```python
from build123d import *

# Parameters (mm, degrees)
BOSS_EXTRUDE1_DEPTH                     = 1247.2780762
BOSS_EXTRUDE1_DEPTH_BACK                = 0.0001
CBORE_FOR_M5_HEX_HEAD_BOLT1_D           = 5.8
CBORE_FOR_M5_HEX_HEAD_BOLT1_CBORE_D     = 12.238
CBORE_FOR_M5_HEX_HEAD_BOLT1_CBORE_DEPTH = 3.5
SKETCH12_R                              = 2.192561761
SKETCH12_R_2                            = 2.198183891
SKETCH12_R_3                            = 2.178555517
SKETCH12_R_4                            = 2.1825859
SKETCH12_R_5                            = 2.191093622
SKETCH12_R_6                            = 2.184131757
SKETCH12_W                              = 20.639060425
SKETCH12_H                              = 4.385123522
SKETCH12_W_2                            = 20.62721893
CUT_EXTRUDE3_DEPTH                      = 219
SCALE1_SCALE                            = 1.8


with BuildPart() as part:
    # Sketch1 → Boss-Extrude1 (new, two sides: drawn at the far end of the back side and taken through both)
    with BuildSketch(Plane.XY.offset(-BOSS_EXTRUDE1_DEPTH_BACK)):
        Polygon((-11.227272727, -5.287267028), (10.772727273, -5.287267028), (10.772727273, 1.712732972), (12.272727273, 1.712732972), (12.272727273, -6.687267028), (-12.727272727, -6.687267028), (-12.727272727, 1.712732972), (-11.227272727, 1.712732972), align=None)
    extrude(amount=BOSS_EXTRUDE1_DEPTH + BOSS_EXTRUDE1_DEPTH_BACK)

    # CBORE for M5 Hex Head Bolt1 (through all)
    with Locations(Plane(origin=(0, -5.287267028, 0), x_dir=(1, 0, 0), z_dir=(0, 1, 0))):
        with Locations((0, -26.226555277), (0, -53.601555277), (0, -80.976555277), (0, -108.351555277), (0, -135.726555277), (0, -163.101555277), (0, -190.476555277), (0, -217.851555277)):
            CounterBoreHole(CBORE_FOR_M5_HEX_HEAD_BOLT1_D / 2, CBORE_FOR_M5_HEX_HEAD_BOLT1_CBORE_D / 2, CBORE_FOR_M5_HEX_HEAD_BOLT1_CBORE_DEPTH)

    # Sketch12 → Cut-Extrude3 (cut)
    with BuildSketch(Plane.ZY.offset(12.727272727)):
        with Locations((13.543356252, -2.543007858)):
            Circle(SKETCH12_R)
        with Locations((34.182416677, -2.543007858)):
            Circle(SKETCH12_R_2)
        with Locations((65.305213992, -2.710382167)):
            Circle(SKETCH12_R)
        with Locations((85.932432922, -2.710382167)):
            Circle(SKETCH12_R_3)
        with Locations((112.703179644, -2.640183104)):
            Circle(SKETCH12_R)
        with Locations((133.330398574, -2.640183104)):
            Circle(SKETCH12_R_4)
        with Locations((164.345985992, -2.803798306)):
            Circle(SKETCH12_R)
        with Locations((184.973204922, -2.803798306)):
            Circle(SKETCH12_R_5)
        with Locations((216.107843732, -2.971172615)):
            Circle(SKETCH12_R)
        with Locations((236.735062662, -2.971172615)):
            Circle(SKETCH12_R_6)
        with Locations((23.862886465, -2.543007858)):
            Rectangle(SKETCH12_W, SKETCH12_H)
        with Locations((75.618823457, -2.710382167)):
            Rectangle(SKETCH12_W_2, SKETCH12_H)
        with Locations((123.016789109, -2.640183104)):
            Rectangle(SKETCH12_W_2, SKETCH12_H)
        with Locations((174.659595457, -2.803798306)):
            Rectangle(SKETCH12_W_2, SKETCH12_H)
        with Locations((226.421453197, -2.971172615)):
            Rectangle(SKETCH12_W_2, SKETCH12_H)
    extrude(amount=-CUT_EXTRUDE3_DEPTH, mode=Mode.SUBTRACT)


with BuildPart() as part_1:
    # Scale1: scaled about (0, 0, 0)
    add(part.part.scale(SCALE1_SCALE))


solid = part_1.part
```
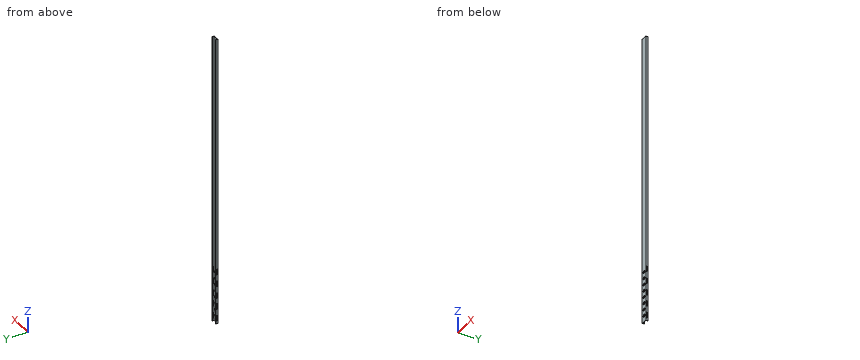
Model file for the job. Use its own axes, mm. Coordinates: 2 decimals unless noted, no trailing zeros. Order: outer loops, then holes, each group sorted by start corner. A loop starts at its lowest first (then second) coordinate and runs counter-clockwise, first axis right, second up. Notation, with made-up numbers: (41.25, 27.5) - (68.25, 27.5) arc R11 cw to (68.25, 37.5) - close; hole circle Ø11 at (-28, 74). An arc over 180 degrees is marked (long way). Return JSON: item names as keys, results as strings. Group by question number.
1) Saw through at A-A, the plane x = 0. Count the separate pieces of the cut face and the enclosed holes in it, plus the area to 3 significant figures.
2) Saw through at B-B, the plane z = 1446.5. Write the cut outline in (x, y), plus the area to 3 significant figures.
3) Probe line 1 (X direction, y = -2, z = 633.5); line 2 (Y direction, x = 9.5, z = 1076). List the from-to ranges inside material, lowest first. Write a range as from..to.
4) Flat gauge pins, fed straight in: P1, Ø1, axis at x = 7.5, z = 2013, coming from the +Y side; P2, Ø8, axis at x = -0.5, y = -6, coming from the -Z side. Where does each tip first touch, or does it go through?
Values found:
{
 "1": {"separate pieces": "9", "enclosed holes": "0", "area": "5,210 mm²"},
 "2": {"outline": "(-22.91, -12.04) - (22.09, -12.04) - (22.09, 3.08) - (19.39, 3.08) - (19.39, -9.52) - (-20.21, -9.52) - (-20.21, 3.08) - (-22.91, 3.08) - close", "area": "181 mm²"},
 "3": {"line 1": "x = -22.91..-20.21, 19.39..22.09", "line 2": "y = -12.04..-9.52"},
 "4": {"P1": "stops at y = -9.52", "P2": "stops at z = 0"}
}
